Autodesk Inventor part; units mm, degrees
ref_plane "Plano de trabajo1" through (18.3204, 15.1618, 2.5684) normal (0, 1, 0) x (-1, 0, 0)
ref_plane "Plano de trabajo2" through (0, 0, 11) normal (0, 0, 1) x (1, 0, 0)
ref_plane "YZ Plane" through (0, 0, 0) normal (1, 0, 0) x (0, 1, 0)
ref_plane "Plano de trabajo1" through (18.3204, 15.1618, 2.5684) normal (0, 1, 0) x (-1, 0, 0)
sketch "Boceto1" plane through (18.3204, 15.1618, 2.5684) normal (0, 1, 0) x (-1, 0, 0)
  circle A0 centre (0, 0) radius 5
  circle A1 centre (0, 0) radius 8
  point P0 (18.3204, -2.5684)
  dimension "d0" = 3
extrude "Extrusión1" add sketch "Boceto1" along normal blind 5 and the other way blind 5
sketch "Boceto2" plane through (18.3204, 20.1618, 2.5684) normal (0, 1, 0) x (1, 0, 0)
  circle A0 centre (0, 0) radius 8
  point P0 (-18.3204, 2.5684)
extrude "Extrusión2" add sketch "Boceto2" along normal blind 5
sketch "Boceto3" plane through (18.3204, 25.1618, 2.5684) normal (0, 1, 0) x (1, 0, 0)
  circle A0 centre (0, 0) radius 2.5
  point P0 (-18.3204, 2.5684)
  dimension "d7" = 5
extrude "Extrusión3" cut sketch "Boceto3" against normal blind 3
ref_plane "Plano de trabajo2" through (0, 0, 11) normal (0, 0, 1) x (1, 0, 0)
sketch "Boceto4" plane through (0, 0, 11) normal (0, 0, 1) x (1, 0, 0)
  line L0 (26.3204, 25.1618) -> (10.3204, 25.1618)
  line L1 (10.3204, 10.1618) -> (26.3204, 10.1618)
  circle A0 centre (18.3204, 15.1618) radius 2.5
  point P0 (0, 0)
  dimension "d11" = 5
  dimension "d12" = 5
extrude "Extrusión4" cut sketch "Boceto4" against normal blind 6
chamfer "Chaflán1" distance 0.5 angle 45 1 edges at (26.3204, 10.1618, 2.5684)
chamfer "Chaflán2" distance 1 angle 45 1 edges at (10.3204, 25.1618, 2.5684)
properties part number "acople_iman"
Input: part model. Units: mm. Frame: model coordinates. A direction names the side the tool comes from. Coordinates: 2 decimals unless noted, no trailing zeros. Loops run counter-clockwise (first coordinate to the right, second up) from the corner with the lowest first, then second, coordinate; pieces in that order, holes last. Notation, with made-up numbers: M 68,59.25 L 88,59.25 A36 ccw 88,96.25 Z; hole C 13,-34.5 d6. An arc over 180 degrees is marked long. Answer in a Markdown table with one row per item.
1. First-contact query: pin 1 (6.5 mm diameter, centred on x = 18.32, z = 2.57, fed in from -Y); pin 2 (4 mm diameter, centred on x = 24, y = 15, fed in from -Z); pin 3 (4 mm diameter, centred on y = 14.5, z = 8.5, fed in from -X). Flat tips, straight axial feed; report the tip coordinate or a pass-through.
Response:
| item | result |
|---|---|
| pin 1 | stops at y = 20.16 |
| pin 2 | stops at z = -4.54 |
| pin 3 | stops at x = 11.35 |
2. Section C-C, the plane y = 18.5. Output: boundary loops of the cut face in (x, z).
Response:
| item | result |
|---|---|
| outline | C 18.32,2.57 d16; hole C 18.32,2.57 d10 |
3. Section D-D, the plane y = 20.75. Output: boundary loops of the cut face in (x, z), then the cut area to 3 significant figures.
Response:
| item | result |
|---|---|
| outline | C 18.32,2.57 d16 |
| area | 201 mm2 |
4. Material intervals for line 1 (Z direction, x = 21.5, y = 15.75); line 2 (X direction, y = 16.25, z = 8.75); line 3 (Y direction, x = 15.75, z = 6), sorted ascending.
Response:
| item | result |
|---|---|
| line 1 | z = -4.77 to -1.29, 6.43 to 9.91 |
| line 2 | x = 13.24 to 16.07, 20.57 to 23.4 |
| line 3 | y = 20.16 to 25.16 |
5. Draft query along X for faces 1 (the flat face through (13, 10.162, 1)), 2 (the flat face through (18, 20.162, 2)), 3 (the cylindrical face through (17.793, 17.317, -5.414)). Return one class per face: pulls with the +X half, pulls with the -X half, needs draft (parallel to the pull), parting line crosses it, or undercut.
Response:
| item | result |
|---|---|
| face 1 | needs draft |
| face 2 | undercut |
| face 3 | parting line crosses it |
6. Section A-A, the plane y = 23.5. Output: boundary loops of the cut face in (x, z).
Response:
| item | result |
|---|---|
| outline | C 18.32,2.57 d16; hole C 18.32,2.57 d5 |
7. Reachability of faces 4 (the cylindrical face through (19.404, 15.232, -2.313)), 5 (the cylindrical face through (20.705, 15.913, 8.76)), 6 (the flat face through (18, 22.162, 3)) from +Z, -Z, +X, -X, +Y, -Y: full face, straight path, thin tool, end or side. Return the list, or none.
Response:
| item | result |
|---|---|
| face 4 | -Y |
| face 5 | +Z |
| face 6 | +Y |
8. Section B-B, the plane y = 14.5. Output: boundary loops of the cut face in (x, z), then the cut area to 3 significant figures.
Response:
| item | result |
|---|---|
| outline | M 15.91,6.95 L 15.91,10.2 A8 ccw long 20.73,10.2 L 20.73,6.95 A5 cw long Z |
| area | 108 mm2 |
